The listing builds one solid part. Answer for the finished solid, in the listing's coordinates (mm). A direction names the side the tool comes from. Coordinates: 2 decimals unless noted, no trailing zeros. Order: outer loops, then holes, each group sorted by start corner. A loop starts at its lowest first (then second) coordinate and runs counter-clockwise, first axis right, second up. Notation, with made-up numbers: (-15.5, -22.75) -> (10.5, -22.75) arc R21 cw to (10.5, -1.75) -> close; hole circle Ø10 at (-22.5, 89). An arc over 180 degrees is marked (long way). One line per question, with ' | ' between items.
from build123d import *

# Parameters (mm, degrees)
BOSS_EXTRUDE1_DEPTH = 3
SKETCH4_R           = 1.25
SKETCH4_R_2         = 2.5
CUT_EXTRUDE1_DEPTH  = 3


with BuildPart() as part:
    # Sketch1 → Boss-Extrude1 (new body)
    with BuildSketch(Plane.XY):
        with BuildLine():
            Line((20.201010127, 40), (-20.201010127, 40))
            Line((-20.201010127, 40), (-107.600505063, 127.399494937))
            ThreePointArc((-107.600505063, 127.399494937), (-127.399494937, 127.399494937), (-127.399494937, 107.600505063))
            Line((-127.399494937, 107.600505063), (-30, 10.201010127))
            Line((-30, 10.201010127), (-30, -10.201010127))
            Line((-30, -10.201010127), (-127.399494937, -107.600505063))
            ThreePointArc((-127.399494937, -107.600505063), (-127.399494937, -127.399494937), (-107.600505063, -127.399494937))
            Line((-107.600505063, -127.399494937), (-20.201010127, -40))
            Line((-20.201010127, -40), (20.201010127, -40))
            Line((20.201010127, -40), (107.600505063, -127.399494937))
            ThreePointArc((107.600505063, -127.399494937), (127.399494937, -127.399494937), (127.399494937, -107.600505063))
            Line((127.399494937, -107.600505063), (30, -10.201010127))
            Line((30, -10.201010127), (30, 10.201010127))
            Line((30, 10.201010127), (127.399494937, 107.600505063))
            ThreePointArc((127.399494937, 107.600505063), (127.399494937, 127.399494937), (107.600505063, 127.399494937))
            Line((107.600505063, 127.399494937), (20.201010127, 40))
        make_face()
    extrude(amount=-BOSS_EXTRUDE1_DEPTH)

    # Sketch4 → Cut-Extrude1 (cut)
    with BuildSketch(Plane.XY):
        with Locations((-108, 117.5)):
            Circle(SKETCH4_R)
        with Locations((-117.5, 108)):
            Circle(SKETCH4_R)
        with Locations((-127, 117.5)):
            Circle(SKETCH4_R)
        with Locations((-117.5, 127)):
            Circle(SKETCH4_R)
        with Locations((-25, 35)):
            Circle(SKETCH4_R_2)
        with Locations((-117.5, -108)):
            Circle(SKETCH4_R)
        with Locations((-127, -117.5)):
            Circle(SKETCH4_R)
        with Locations((-117.5, -127)):
            Circle(SKETCH4_R)
        with Locations((-108, -117.5)):
            Circle(SKETCH4_R)
        with Locations((-25, -35)):
            Circle(SKETCH4_R_2)
        with Locations((108, -117.5)):
            Circle(SKETCH4_R)
        with Locations((117.5, -127)):
            Circle(SKETCH4_R)
        with Locations((127, -117.5)):
            Circle(SKETCH4_R)
        with Locations((117.5, -108)):
            Circle(SKETCH4_R)
        with Locations((117.5, 108)):
            Circle(SKETCH4_R)
        with Locations((127, 117.5)):
            Circle(SKETCH4_R)
        with Locations((117.5, 127)):
            Circle(SKETCH4_R)
        with Locations((108, 117.5)):
            Circle(SKETCH4_R)
        with Locations((25, -35)):
            Circle(SKETCH4_R_2)
        with Locations((25, 35)):
            Circle(SKETCH4_R_2)
    extrude(amount=-CUT_EXTRUDE1_DEPTH, mode=Mode.SUBTRACT)


solid = part.part
Item 1: Determine the mould class of faces 1 (the face through (-1, 10, 0)), 2 (the face through (-79.4, 59.6, -1.5)), 3 (the face through (78, 58.2, -1.5)), 4 (the face through (-64.5, -84.3, -1.5)) for opening direction X: pulls with the +X half, pulls with the -X half, needs draft (parallel to the pull), parting line crosses it, or undercut.
Computed values:
face 1: needs draft | face 2: pulls with the -X half | face 3: pulls with the +X half | face 4: undercut
Item 2: For faces 5 (the face through (64.5, 84.3, -1.5)), 6 (the face through (63.3, -83.1, -1.5)), 7 (the face through (-78, -58.2, -1.5)), 8 (the face through (79.4, -59.6, -1.5)), determine the directions among +Z, -Z, +X, -X, +Y, -Y from which every point of the face is accessible in a straight line to the end or side of a thin tool.
Computed values:
face 5: +Z, -Z, +Y | face 6: +Z, -Z, -Y | face 7: +Z, -Z, -X | face 8: +Z, -Z, +X
Item 3: Section B-B, the plane z = -1.8 is taken. Count the separate pieces of the cut face and the enclosed holes in it, plus the area to 3 significant figures.
Computed values:
separate pieces: 1 | enclosed holes: 20 | area: 19,900 mm^2
Item 4: Find the intervals of material crossed by L1, parallel to X at y = 108.5, z = -0.9; L2, parallel to X at y = -117.5, z = -2, in increasing order.
Computed values:
L1: x = -128.22 to -118.65, -116.35 to -88.7, 88.7 to 116.35, 118.65 to 128.22 | L2: x = -131.5 to -128.25, -125.75 to -109.25, -106.75 to -97.7, 97.7 to 106.75, 109.25 to 125.75, 128.25 to 131.5
Item 5: Section A-A, the plane y = 44.5 is taken. Give the vertices of the cut face in (x, z).
Computed values:
outline: (-64.3, -3) -> (-24.7, -3) -> (-24.7, 0) -> (-64.3, 0) -> close; (24.7, -3) -> (64.3, -3) -> (64.3, 0) -> (24.7, 0) -> close
Item 6: Each of these flat-tipped pins is pushed along its axis until it touches: pin 1 Ø1.5 at (x, z) = (3, -1) entering from +Y; pin 2 Ø1 at (y, z) = (85, -2) entering from -X; pin 3 Ø1.5 at (y, z) = (4.5, -1.5) entering from +X. Where does it stop, or does it pass through?
Computed values:
pin 1: stops at y = 40 | pin 2: stops at x = -105.3 | pin 3: stops at x = 30
